```python
from build123d import *

# Parameters (mm, degrees)
FILLET3_R           = 100
CUT_EXTRUDE2_DEPTH  = 616.4266812545585
CUT_EXTRUDE3_DEPTH  = 606.1859218455102
CUT_EXTRUDE18_DEPTH = 595.7688626685159


with BuildPart() as part:
    # Sweep1: sweep along a path in Sketch3
    with BuildLine(Plane(origin=(0, 0, 0), x_dir=(0, 0, -1), z_dir=(1, 0, 0))) as sweep1_path:
        Line((0, 0), (0, 500))
        Line((0, 500), (250, 500))
        Line((250, 500), (250.00000000000006, 6.12e-15))
        Line((250.00000000000006, 6.12e-15), (0, 0))
    # Sketch2 → Sweep1 (sweep)
    with BuildSketch(Plane(origin=(0, 0, 0), x_dir=(1, 0, 0), z_dir=(0, 1, 0))):
        Polygon((25, -25), (-25, -25.00000000000001), (-25, 24.999999999999993), (25, 24.999999999999996), align=None)
        Polygon((20, 19.999999999999996), (-20, 19.99999999999999), (-20, -20.000000000000007), (20, -20), align=None, mode=Mode.SUBTRACT)
    sweep(path=sweep1_path.line, transition=Transition.RIGHT)

    # Fillet3
    fillet3_edges = [part.edges().sort_by_distance(p)[0] for p in [
        (0, 25, -225),
        (0, 25, -24.999999999999996),
        (0, 475, -225),
        (0, 475, -24.999999999999996),
    ]]
    fillet(fillet3_edges, radius=FILLET3_R - 0.0001)  # a hair under: the kernel refuses the full size
    fillet3_2_edges = [part.edges().sort_by_distance(p)[0] for p in [
        (-3.55e-15, 525, -275),
        (-3.55e-15, -25.000000000000004, -275),
        (-3.55e-15, -25.00000000000001, 25.000000000000007),
        (-3.55e-15, 525, 25.000000000000007),
    ]]
    fillet(fillet3_2_edges, radius=FILLET3_R)

    # Sketch5 → Cut-Extrude2 (cut, through all)
    with BuildSketch(Plane.XZ.offset(25.000000000000014)):
        Polygon((-20.000000000000007, -170.00000000000006), (19.999999999999993, -170.00000000000006), (19.999999999999993, -79.99999999999999), (-20.000000000000007, -79.99999999999996), align=None)
    extrude(amount=-CUT_EXTRUDE2_DEPTH, mode=Mode.SUBTRACT)

    # Sketch6 → Cut-Extrude3 (cut, through all)
    with BuildSketch(Plane.XY.offset(25.000000000000007)):
        Polygon((-20.000000000000007, 420.00000000000006), (-20.000000000000007, 79.99999999999997), (19.999999999999993, 79.99999999999999), (19.999999999999993, 420.00000000000006), align=None)
    extrude(amount=-CUT_EXTRUDE3_DEPTH, mode=Mode.SUBTRACT)

    # Sketch19 → Cut-Extrude18 (cut, through all)
    with BuildSketch(Plane.ZY.offset(25)):
        with BuildLine():
            ThreePointArc((-224.89347851891705, 421.05749612593655), (-232.44366579068512, 398.57665543412725), (-235.00000000000003, 375))
            Line((-235.00000000000003, 375), (-235.00000000000006, 125))
            ThreePointArc((-235.00000000000006, 125), (-232.44366579068517, 101.42334456587275), (-224.89347851891705, 78.94250387406343))
            Line((-224.89347851891705, 78.94250387406343), (-265.0000000000001, 74.99999999999996))
            Line((-265.0000000000001, 74.99999999999996), (-265, 425.00000000000006))
            Line((-265, 425.00000000000006), (-224.89347851891705, 421.05749612593655))
        make_face()
        with BuildLine():
            ThreePointArc((-238.63961030678925, 488.63961030678945), (-256.1053768922045, 464.0117653942177), (-264.44344676082267, 434.9934894578369))
            Line((-264.44344676082267, 434.9934894578369), (-219.90488415304466, 430.61531231501976))
            ThreePointArc((-219.90488415304463, 430.61531231501976), (-212.0517417816099, 442.2457749809452), (-202.7817459305202, 452.78174593052023))
            Line((-202.7817459305202, 452.78174593052023), (-238.63961030678934, 488.6396103067894))
        make_face()
        with BuildLine():
            ThreePointArc((-184.1609145540828, 514.532550754085), (-213.63405487722474, 506.2859754431452), (-238.63961030678925, 488.63961030678945))
            Line((-238.63961030678934, 488.6396103067894), (-202.7817459305202, 452.78174593052023))
            ThreePointArc((-202.78174593052017, 452.78174593052023), (-192.16702134643737, 462.1125205894492), (-180.4435650027513, 470.00532142877944))
            Line((-180.4435650027513, 470.00532142877944), (-184.1609145540828, 514.532550754085))
        make_face()
        with BuildLine():
            ThreePointArc((-79.17424305044158, 475), (-101.54792120088285, 482.4709263010234), (-125, 485))
            ThreePointArc((-125, 485), (-148.45207879911717, 482.4709263010234), (-170.82575694955844, 475))
            Line((-170.82575694955844, 475), (-174.16515138991173, 515))
            Line((-174.16515138991173, 515), (-75.83484861008839, 515))
            Line((-75.83484861008839, 515), (-79.17424305044158, 475))
        make_face()
        with BuildLine():
            Line((-47.21825406947977, 452.7817459305203), (-11.360389693210657, 488.6396103067894))
            ThreePointArc((-11.36038969321067, 488.6396103067894), (-36.365945122775244, 506.2859754431452), (-65.83908544591725, 514.532550754085))
            Line((-65.83908544591723, 514.532550754085), (-69.55643499724876, 470.00532142877944))
            ThreePointArc((-69.55643499724874, 470.00532142877944), (-57.83297865356265, 462.11252058944933), (-47.21825406947981, 452.78174593052034))
        make_face()
        with BuildLine():
            Line((-30.0951158469554, 430.61531231501976), (14.443446760822598, 434.9934894578369))
            ThreePointArc((14.443446760822624, 434.9934894578369), (6.105376892204447, 464.0117653942176), (-11.36038969321067, 488.6396103067894))
            Line((-11.360389693210657, 488.6396103067894), (-47.21825406947977, 452.7817459305203))
            ThreePointArc((-47.21825406947981, 452.78174593052034), (-37.94825821839011, 442.24577498094527), (-30.09511584695541, 430.61531231501976))
        make_face()
        with BuildLine():
            ThreePointArc((-25.106521481082943, 78.94250387406343), (-17.556334209314883, 101.42334456587272), (-15.000000000000027, 125))
            Line((-15.000000000000027, 125), (-14.999999999999995, 375))
            ThreePointArc((-14.999999999999995, 375), (-17.556334209314898, 398.57665543412725), (-25.106521481082943, 421.05749612593655))
            Line((-25.106521481082943, 421.05749612593655), (15.00000000000007, 425.00000000000006))
            Line((15.00000000000007, 425.00000000000006), (15.000000000000012, 74.99999999999997))
            Line((15.000000000000012, 74.99999999999997), (-25.106521481082943, 78.94250387406343))
        make_face()
        with BuildLine():
            Line((14.443446760822598, 65.00651054216311), (-30.0951158469554, 69.38468768498025))
            ThreePointArc((-30.0951158469554, 69.38468768498025), (-37.948258218390094, 57.754225019054786), (-47.2182540694798, 47.218254069479784))
            ThreePointArc((-47.2182540694798, 47.218254069479784), (-57.832978653562634, 37.887479410550725), (-69.55643499724876, 29.994678571220568))
            Line((-69.55643499724876, 29.994678571220568), (-65.83908544591723, -14.532550754084966))
            ThreePointArc((-65.83908544591723, -14.532550754084966), (-36.36594512277525, -6.285975443145162), (-11.360389693210696, 11.360389693210667))
            ThreePointArc((-11.360389693210696, 11.360389693210667), (6.105376892204447, 35.98823460578241), (14.443446760822598, 65.00651054216311))
        make_face()
        with BuildLine():
            ThreePointArc((-125.00000000000003, 15), (-101.54792120088285, 17.529073698976617), (-79.17424305044158, 25.00000000000002))
            Line((-79.17424305044158, 25.00000000000002), (-75.8348486100883, -15.00000000000004))
            Line((-75.8348486100883, -15.00000000000004), (-174.16515138991173, -15.000000000000016))
            Line((-174.16515138991173, -15.000000000000016), (-170.82575694955844, 25.00000000000002))
            ThreePointArc((-170.82575694955844, 25.00000000000002), (-148.45207879911717, 17.52907369897663), (-125.00000000000003, 15))
        make_face()
        with BuildLine():
            ThreePointArc((-264.44344676082267, 65.00651054216311), (-256.1053768922045, 35.9882346057824), (-238.63961030678936, 11.360389693210667))
            ThreePointArc((-238.63961030678936, 11.360389693210667), (-213.6340548772248, -6.285975443145162), (-184.1609145540828, -14.532550754084966))
            Line((-184.1609145540828, -14.532550754084966), (-180.4435650027513, 29.994678571220568))
            ThreePointArc((-180.4435650027513, 29.994678571220568), (-192.16702134643742, 37.88747941055071), (-202.7817459305203, 47.218254069479755))
            ThreePointArc((-202.7817459305203, 47.218254069479755), (-212.05174178160996, 57.754225019054815), (-219.90488415304466, 69.38468768498025))
            Line((-219.90488415304466, 69.38468768498025), (-264.44344676082267, 65.00651054216311))
        make_face()
    extrude(amount=-CUT_EXTRUDE18_DEPTH, mode=Mode.SUBTRACT)


solid = part.part
```
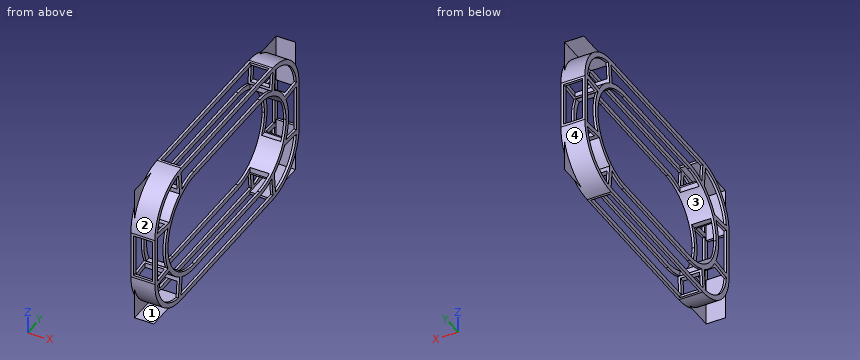
For this review, take the finished solid that the model builds, in its own axes (mm). Face numbers are marked on the shaded views. A direction names the side the tool comes from. Round coordinates to 2 decimals unless told otherwise and drop trailing zeros. Order: outer loops, then holes, each group sorted by start corner. A loop starts at its lowest first (then second) coordinate and runs counter-clockwise, first axis right, second up. Notation, with made-up numbers: (83, -8) -> (136, -8) arc R21 ccw to (136, 11) -> close; hole circle Ø1 at (34.25, 87). An arc over 180 degrees is marked (long way). Use a Markdown table: item, result.
Item 1: Draft analysis for pull direction Z (two halves, no side actions). For the marked faces 1 and 2, state which applies: +Z half, -Z half, draft (parallel to the pull), parting line (faces both ways), or undercut.
Resolved:
| item | result |
|---|---|
| face 1 | undercut |
| face 2 | undercut |
Item 2: For pin 1 (12 mm diameter, centred on x = 11.5, y = 427, fed in from -Z); pin 2 (6 mm diameter, centred on x = 18.5, z = -182.5, fed in from +Y); pin 3 (5 mm diameter, centred on x = 1, y = 431, fed in from +Z); pin 4 (1.5 mm diameter, centred on x = 13, z = -55.5, fed in from +Y), all flat-tipped, find the tip position at first contact; note any pin that passes through.
Resolved:
| item | result |
|---|---|
| pin 1 | stops at z = -275 |
| pin 2 | stops at y = 524.9 |
| pin 3 | stops at z = 24.94 |
| pin 4 | stops at y = 523.23 |
Item 3: Take a section at D-D (z = -53). State the section outline as (x, y) points, plus the area to 3 significant figures.
Resolved:
| item | result |
|---|---|
| outline | (-25, -22.55) -> (25, -22.55) -> (25, -12.27) -> (20, -12.27) -> (20, -20) -> (-20, -20) -> (-20, -12.27) -> (-25, -12.27) -> close; (-25, 41.84) -> (25, 41.84) -> (25, 55.6) -> (-25, 55.6) -> close; (-25, 444.4) -> (25, 444.4) -> (25, 458.16) -> (-25, 458.16) -> close; (-25, 512.27) -> (-20, 512.27) -> (-20, 520) -> (20, 520) -> (20, 512.27) -> (25, 512.27) -> (25, 522.55) -> (-25, 522.55) -> close |
| area | 1,790 mm² |
Item 4: For line 1 along Z through (x, y) = (-21.5, 349); line 2 along Y through (x, z) = (23, -115); line 3 along Z through (x, y) = (-23, 386), list the stretches that pass through material, from the lowest coordinate up. Write a range as [from, to].
Resolved:
| item | result |
|---|---|
| line 1 | z = [-275, -265], [-235, -225], [-25, -15], [15, 25] |
| line 2 | y = [-25, -15], [15.46, 25.5], [474.5, 484.54], [515, 525] |
| line 3 | z = [-275, -265], [-234.45, -224.39], [-25.61, -15.55], [15, 25] |
Item 5: Machinability: for the marked faces 3 and 4, which of the approach directions +Z, -Z, +X, -X, +Y, -Y give a long, thin tool a straight path to every point of the face, cutting with its end or side? Answer none if there is none.
Resolved:
| item | result |
|---|---|
| face 3 | +X, -X |
| face 4 | none |
Item 6: Take a section at A-A (y = 231). State how many separate pieces and enclosed holes the cut face has, plus the area to 3 significant figures.
Resolved:
| item | result |
|---|---|
| separate pieces | 8 |
| enclosed holes | 0 |
| area | 400 mm² |
